Source: CAD feature listing. Evaluate the final solid. Frame: model axes, mm. Give positions to 0.01 mm unless a question says otherwise; leave off trailing zeros. Write each loop counter-clockwise with the first axis right and the second up, starting at its lowest first coordinate (ties: lowest second). Pieces come first, ordered by that corner, then holes.
```python
from build123d import *

# Parameters (mm, degrees)
MODEL_R                     = 15
MODEL_R_2                   = 2.6
BASE_DEPTH                  = 6
SKETCH2_R                   = 2
CABLETIEMOUNT_DEPTH         = 7
F_3_5_3_5_STEPPERMOUNT_D    = 3.5
F_3_5_3_5_CABLECHAINMOUNT_D = 3.5


with BuildPart() as part:
    # Model → Base (new body)
    with BuildSketch(Plane.XY):
        with BuildLine():
            Line((47, 98), (47, 12))
            ThreePointArc((47, 12), (43.485281374, 3.514718626), (35, 0))
            Line((35, 0), (-35, 0))
            ThreePointArc((-35, 0), (-43.485281374, 3.514718626), (-47, 12))
            Line((-47, 12), (-47, 98))
            ThreePointArc((-47, 98), (-43.485281374, 106.485281374), (-35, 110))
            Line((-35, 110), (35, 110))
            ThreePointArc((35, 110), (43.485281374, 106.485281374), (47, 98))
        make_face()
        with Locations((0, 25)):
            Circle(MODEL_R, mode=Mode.SUBTRACT)
        with Locations((27, 98.3)):
            Circle(MODEL_R_2, mode=Mode.SUBTRACT)
        with Locations((-27, 98.3)):
            Circle(MODEL_R_2, mode=Mode.SUBTRACT)
        with BuildLine():
            Line((-29.6, 40.1), (-29.6, 37.6))
            ThreePointArc((-29.6, 37.6), (-27, 35), (-24.4, 37.6))
            Line((-24.4, 37.6), (-24.4, 40.1))
            ThreePointArc((-24.4, 40.1), (-27, 42.7), (-29.6, 40.1))
        make_face(mode=Mode.SUBTRACT)
        with BuildLine():
            Line((29.6, 37.6), (29.6, 40.1))
            ThreePointArc((29.6, 40.1), (27, 42.7), (24.4, 40.1))
            Line((24.4, 40.1), (24.4, 37.6))
            ThreePointArc((24.4, 37.6), (27, 35), (29.6, 37.6))
        make_face(mode=Mode.SUBTRACT)
    extrude(amount=BASE_DEPTH)

    # Sketch2 → CableTieMount (cut, through all)
    with BuildSketch(Plane.XY.offset(6)):
        with Locations((31.5, 5.5)):
            Circle(SKETCH2_R)
    extrude(amount=-CABLETIEMOUNT_DEPTH, mode=Mode.SUBTRACT)

    # Ø3.5 (3.5) StepperMount (through all)
    with Locations(Plane.XY.offset(6)):
        with Locations((-15.5, 40.5), (-15.5, 9.5), (15.5, 9.5), (15.5, 40.5)):
            Hole(F_3_5_3_5_STEPPERMOUNT_D / 2)

    # Ø3.5 (3.5) CableChainMount (through all)
    with Locations(Plane(origin=(0, 0, 0), x_dir=(-1, 0, 0), z_dir=(0, 0, -1))):
        with Locations((-37.5, 58), (-29, 58)):
            Hole(F_3_5_3_5_CABLECHAINMOUNT_D / 2)


solid = part.part
```
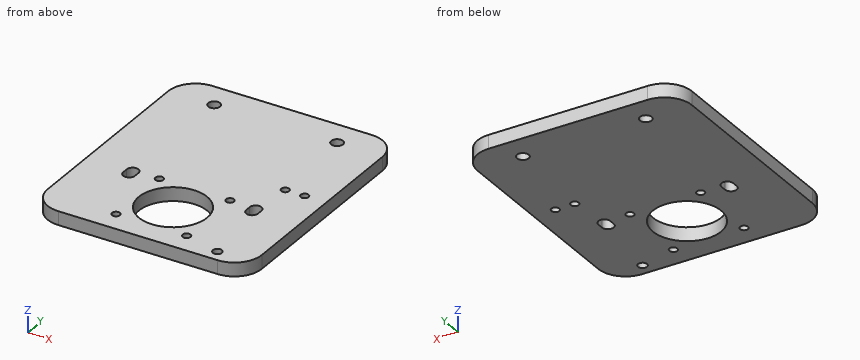
1. Cut plane C-C, the plane x = -27. Return the cut outline in (y, z).
2. Cut plane A-A, the plane x = 0. Return the cut outline in (y, z), then the cut area to 3 significant figures.
3. Cut plane D-D, the plane z = 1.4. State how many separate pieces and enclosed holes the cut face has, then the cut area to 3 significant figures.
4. Line query: L1, parallel to Y at x = -15.5, z = 1.3; L2, parallel to Y at x = 31.5, z = 2.9; L3, parallel to Y at x = 0, z = 3.9. Output: solid intervals per line, ascending.
5. Cut plane B-B, the plane y = 58. Return the cut outline in (x, z), then the cut area to 3 significant figures.
Response values:
1. outline: (0, 0) - (35, 0) - (35, 6) - (0, 6) - close; (42.7, 0) - (95.7, 0) - (95.7, 6) - (42.7, 6) - close; (100.9, 0) - (110, 0) - (110, 6) - (100.9, 6) - close
2. outline: (0, 0) - (10, 0) - (10, 6) - (0, 6) - close; (40, 0) - (110, 0) - (110, 6) - (40, 6) - close
2. area: 480 mm2
3. separate pieces: 1
3. enclosed holes: 12
3. area: 9,330 mm2
4. L1: y = 0 to 7.75, 11.25 to 38.75, 42.25 to 110
4. L2: y = 0 to 3.5, 7.5 to 110
4. L3: y = 0 to 10, 40 to 110
5. outline: (-47, 0) - (27.25, 0) - (27.25, 6) - (-47, 6) - close; (30.75, 0) - (35.75, 0) - (35.75, 6) - (30.75, 6) - close; (39.25, 0) - (47, 0) - (47, 6) - (39.25, 6) - close
5. area: 522 mm2
